from build123d import *

# Parameters (mm, degrees)
SKETCH1_R           = 8
SKETCH1_R_2         = 4
BOSS_EXTRUDE1_DEPTH = 8
SKETCH4_R           = 2.5
CUT_EXTRUDE1_DEPTH  = 8
FILLET1_R           = 0.5


with BuildPart() as part:
    # Sketch1 → Boss-Extrude1 (new body)
    with BuildSketch(Plane(origin=(0, 0, 0), x_dir=(1, 0, 0), z_dir=(0, 1, 0))):
        with Locations(Location((0, 0, 0), (0, 0, 270))):
            Circle(SKETCH1_R)
        with Locations(Location((0, 0, 0), (0, 0, 270))):
            Circle(SKETCH1_R_2, mode=Mode.SUBTRACT)
    extrude(amount=BOSS_EXTRUDE1_DEPTH)

    # Sketch4 → Cut-Extrude1 (cut)
    with BuildSketch(Plane(origin=(0, 0, 0), x_dir=(0, 0, -1), z_dir=(1, 0, 0))):
        with Locations((0, 4)):
            Circle(SKETCH4_R)
    extrude(amount=-CUT_EXTRUDE1_DEPTH, mode=Mode.SUBTRACT)

    # Fillet1
    fillet1_edges = [part.edges().sort_by_distance(p)[0] for p in [
        (0, 0, -8),
        (0, 8, -8),
        (0, 0, -4),
        (0, 8, -4),
    ]]
    fillet(fillet1_edges, radius=FILLET1_R)


solid = part.part
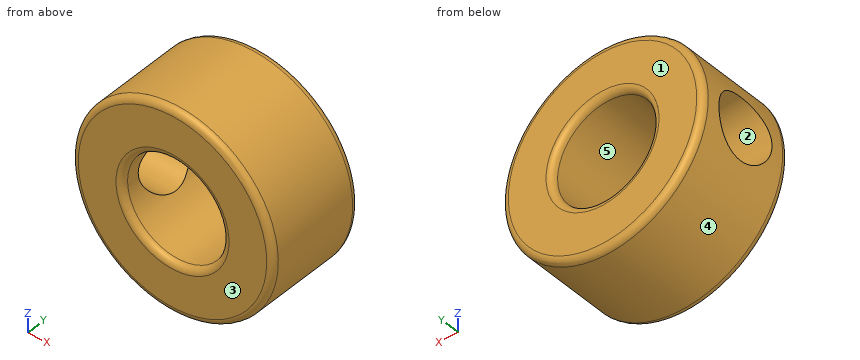
Design review of the part built by this model. Coordinates are the model's own, in mm. Face numbers are marked on the shaded views. A direction names the side the tool comes from. Round coordinates to 2 decimals unless told otherwise and drop trailing zeros. Write each loop counter-clockwise with the first axis right and the second up, starting at its lowest first coordinate (ties: lowest second). Pieces come first, ordered by that corner, then holes. Notation, with made-up numbers: (65.25, -11.5) -> (112.25, -11.5) arc R28 ccw to (112.25, 27.5) -> close; hole circle Ø10 at (63.25, 87). An arc over 180 degrees is marked (long way). One line per item, written item: value. Start each with the question number.
Q1. Add section C-C (y = 1). Give the boundary of the cut face in (x, z), then the cut area to 3 significant figures.
Q2. Tool access review of the marked faces 1 and 2: name each direction out of +Z, -Z, +X, -X, +Y, -Y from which nothing blocks a thin tool from reaching the whole face with its end or side.
Q3. The part is to be moulded in two halves that separate along X. For the marked faces 3, 4 and 5, say which applies: pulls with the +X half, pulls with the -X half, needs draft (parallel to the pull), parting line crosses it, or undercut.
Q4. To check wall thickness, follow probe 1 along Y at (x, z) = (-6.05, 0); probe 2 along X at (y, z) = (5.5, 0); probe 3 along Z at (x, y) = (-4.6, 4). State the ranges of each line that lie inside material, in increasing order.
Q5. Add section B-B (x = 0). Give the boundary of the cut face in (y, z).
Q6. Add section D-D (y = 5.75). Give the boundary of the cut face in (x, z), then the cut area to 3 significant figures.
Q7. Insertion check: P1, Ø4, axis at x = 5, y = 1, coming from the -Z side; P2, Ø3, axis at x = -5.5, y = 6, coming from the +Z side; P3, Ø3, axis at y = 4, z = 0, coming from the -X side. Each pin has a flat end and moves straight along its axis. Give the tip position at first contact, or say it passes through.
Q8. Add section A-A (z = 0). Give the boundary of the cut face in (x, y).
Response:
1. outline: circle Ø16 at (0, 0); hole circle Ø8 at (0, 0)
1. area: 151 mm^2
2. face 1: +Z, -Z, +X, -X, +Y
2. face 2: -X
3. face 3: needs draft
3. face 4: parting line crosses it
3. face 5: undercut
4. probe 1: y = 0 to 1.5, 6.5 to 8
4. probe 2: x = 4 to 8
4. probe 3: z = -6.55 to -2.5, 2.5 to 6.55
5. outline: (0, -7.5) arc R0.5 ccw to (0.5, -8) -> (7.5, -8) arc R0.5 ccw to (8, -7.5) -> (8, -4.5) arc R0.5 ccw to (7.5, -4) -> (0.5, -4) arc R0.5 ccw to (0, -4.5) -> close; (0, 4.5) arc R0.5 ccw to (0.5, 4) -> (7.5, 4) arc R0.5 ccw to (8, 4.5) -> (8, 7.5) arc R0.5 ccw to (7.5, 8) -> (0.5, 8) arc R0.5 ccw to (0, 7.5) -> close
6. outline: (-7.8, -1.79) arc R8 ccw (long way) to (-7.8, 1.79) -> (-3.58, 1.79) arc R4 cw (long way) to (-3.58, -1.79) -> close
6. area: 136 mm^2
7. P1: stops at z = -7.42
7. P2: stops at z = 6.93
7. P3: stops at x = 3.71
8. outline: (-8, 0.5) arc R0.5 ccw to (-7.5, 0) -> (-4.5, 0) arc R0.5 ccw to (-4, 0.5) -> (-4, 1.5) -> (-8, 1.5) -> close; (-8, 6.5) -> (-4, 6.5) -> (-4, 7.5) arc R0.5 ccw to (-4.5, 8) -> (-7.5, 8) arc R0.5 ccw to (-8, 7.5) -> close; (4, 0.5) arc R0.5 ccw to (4.5, 0) -> (7.5, 0) arc R0.5 ccw to (8, 0.5) -> (8, 7.5) arc R0.5 ccw to (7.5, 8) -> (4.5, 8) arc R0.5 ccw to (4, 7.5) -> close
